from build123d import *

# Parameters (mm, degrees)
F0_R     = 3
F1_DEPTH = 1
F2_R     = 2.5
F3_DEPTH = 6
F4_R     = 2.5
F5_W     = 2.035479
F5_H     = 6.262277
F5_W_2   = 2.073893
F5_H_2   = 6.24879
F6_DEPTH = 12.5
F7_R     = 1
F8_DEPTH = 25


with BuildPart() as f1:
    # F0 (on Top) → F1 (new body)
    with BuildSketch(Plane.XY):
        Circle(F0_R)
    extrude(amount=F1_DEPTH)

    # F2 (on face) → F3 (join)
    with BuildSketch(Plane.XY.offset(1)):
        Circle(F2_R)
    extrude(amount=F3_DEPTH)

    # F4
    f4_edges = [f1.edges().sort_by_distance(p)[0] for p in [
        (-2.5, 0, 7),
    ]]
    fillet(f4_edges, radius=F4_R)

    # F5 (on Front) → F6 (cut, symmetric)
    with BuildSketch(Plane.XZ):
        with Locations((2.01774, 4.131139)):
            Rectangle(F5_W, F5_H)
        with Locations((-2.036946, 4.124395)):
            Rectangle(F5_W_2, F5_H_2)
    extrude(amount=F6_DEPTH, both=True, mode=Mode.SUBTRACT)

    # F7 (on face) → F8 (cut)
    with BuildSketch(Plane(origin=(-1, 0, 0), x_dir=(0, -1, 0), z_dir=(-1, 0, 0))):
        with Locations((0, 4.5)):
            Circle(F7_R)
    extrude(amount=-F8_DEPTH, mode=Mode.SUBTRACT)


solid = f1.part
Here's how the part is built. I have some questions about the finished solid (model axes, mm). A direction names the side the tool comes from. Give positions to 0.01 mm unless a question says otherwise; leave off trailing zeros. Order: outer loops, then holes, each group sorted by start corner. A loop starts at its lowest first (then second) coordinate and runs counter-clockwise, first axis right, second up. Notation, with made-up numbers: M 19.25,71 L 52.25,71 A24 cw 52.25,85 Z; hole C 54,42.5 d6. An arc over 180 degrees is marked long. Answer as a JSON object with one key per item and string values. Group by question number.
1) Suppose I cut it at C-C, the plane z = 5.25. Write out the boundary of the cut face in (x, y).
2) I'm going to push flat-ended pins straight in: pin 1 Ø1.8 at (y, z) = (0, 4.5) entering from -X; pin 2 Ø3 at (x, y) = (-0.5, -2) entering from +Z; pin 3 Ø1 at (x, y) = (2.5, -1.5) entering from -Z; pin 4 Ø3.5 at (y, z) = (0.5, 3.5) entering from +X. Where does each tip first touch, or does it pass through?
3) Suppose I cut it at A-A, the plane x = 0. Write out the boundary of the cut face in (y, z).
4) Please list where these lines run through material, in increasing order: L1, parallel to Z at x = 0.35, y = 0; L2, parallel to X at y = -1.85, z = 5.25; L3, parallel to Y at x = 0.85, z = 4.25. Write a range as [from, to].
5) Suppose I cut it at D-D, the plane z = 2. Write out the boundary of the cut face in (x, y).
6) On a 3-axis mill with a long thin cutter (end or side, diameter ignored), from which of +Z, -Z, +X, -X, +Y, -Y can I reach the whole of each face in a straight line? I mean faces 1 (the flat face through (2, 0, 1)), 2 (the cylindrical face through (0.31, -2.48, 2.73)), 3 (the cylindrical face through (-0.168, 2.494, 2.726)). Say none if no direction works.
7) We'd pull the mould along Z, two halves only. Please class faces 4 (the flat face through (-1, 0, 3)), 5 (the cylindrical face through (-0.01, 0.13, 5.49)), 6 (the flat face through (0, 0, 0)): pulls with the +Z half, pulls with the -Z half, needs draft (parallel to the pull), parting line crosses it, or undercut.
8) Suppose I cut it at B-B, the plane y = 0.5. Write out the boundary of the cut face in (x, z), plus the area to 3 significant figures.
Results found:
{
 "1": {"outline": "M -1,-2.17 A2.38 ccw 1,-2.17 L 1,-0.66 L -1,-0.66 Z; M -1,0.66 L 1,0.66 L 1,2.17 A2.38 ccw -1,2.17 Z"},
 "2": {"pin 1": "through", "pin 2": "z = 6.94", "pin 3": "z = 0", "pin 4": "x = 1"},
 "3": {"outline": "M -3,0 L 3,0 L 3,1 L 2.5,1 L 2.5,4.5 A2.5 ccw -2.5,4.5 L -2.5,1 L -3,1 Z; hole C 0,4.5 d2"},
 "4": {"L1": "[0, 3.5], [5.5, 6.98]", "L2": "[-1, 1]", "L3": "[-2.35, -0.97], [0.97, 2.35]"},
 "5": {"outline": "M -1,-2.29 A2.5 ccw 1,-2.29 L 1,2.29 A2.5 ccw -1,2.29 Z"},
 "6": {"face 1": "+Z, +X, +Y, -Y", "face 2": "+Z, -Y", "face 3": "+Z, +Y"},
 "7": {"face 4": "needs draft", "face 5": "undercut", "face 6": "pulls with the -Z half"},
 "8": {"outline": "M -2.96,0 L 2.96,0 L 2.96,1 L 1,1 L 1,3.63 L -1,3.63 L -1,1 L -2.96,1 Z; M -1,5.37 L 1,5.37 L 1,6.74 A2.45 ccw -1,6.74 Z", "area": "14.2 mm²"}
}
